from build123d import *

# Parameters (mm, degrees)
F0_R     = 1.5
F0_R_2   = 19
F0_R_3   = 17.5
F1_DEPTH = 2
F2_SIZE  = 1
F3_SIZE  = 1.5


with BuildPart() as f1:
    # F0 (on Top) → F1 (new body)
    with BuildSketch(Plane.XY):
        with BuildLine():
            Line((-22.3, 19.5), (-22.3, -19.5))
            ThreePointArc((-22.3, -19.5), (-21.4798989873, -21.4798989873), (-19.5, -22.3))
            Line((-19.5, -22.3), (19.5, -22.3))
            ThreePointArc((19.5, -22.3), (21.4798989873, -21.4798989873), (22.3, -19.5))
            Line((22.3, -19.5), (22.3, 19.5))
            ThreePointArc((22.3, 19.5), (21.4798989873, 21.4798989873), (19.5, 22.3))
            Line((19.5, 22.3), (-19.5, 22.3))
            ThreePointArc((-19.5, 22.3), (-21.4798989873, 21.4798989873), (-22.3, 19.5))
        make_face()
        with Locations((-19.5, -19.5)):
            Circle(F0_R, mode=Mode.SUBTRACT)
        with Locations((19.5, -19.5)):
            Circle(F0_R, mode=Mode.SUBTRACT)
        with Locations((-19.5, 19.5)):
            Circle(F0_R, mode=Mode.SUBTRACT)
        Circle(F0_R_2, mode=Mode.SUBTRACT)
        with Locations((19.5, 19.5)):
            Circle(F0_R, mode=Mode.SUBTRACT)
        Circle(F0_R_2)
        Circle(F0_R_3, mode=Mode.SUBTRACT)
    extrude(amount=F1_DEPTH)

    # F2
    f2_edges = [f1.edges().sort_by_distance(p)[0] for p in [
        (-21, 19.5, 2),
        (18, 19.5, 2),
        (18, -19.5, 2),
        (-21, -19.5, 2),
    ]]
    chamfer(f2_edges, length=F2_SIZE)

    # F3
    f3_edges = [f1.edges().sort_by_distance(p)[0] for p in [
        (-17.5, 0, 0),
    ]]
    chamfer(f3_edges, length=F3_SIZE)


solid = f1.part
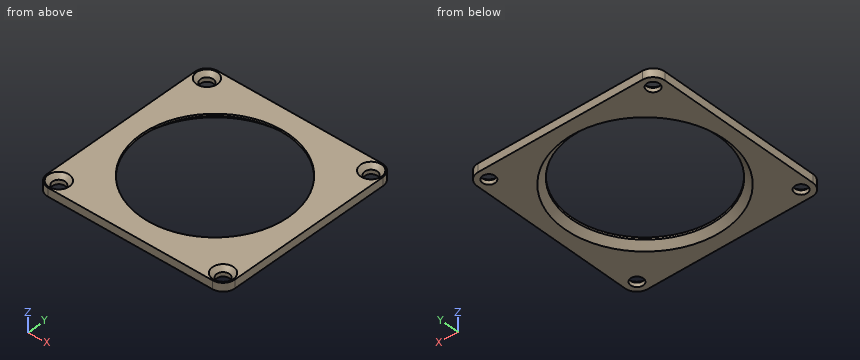
For this review, take the finished solid that the model builds, in its own axes (mm). Coordinates: 2 decimals unless noted, no trailing zeros. Loops run counter-clockwise (first coordinate to the right, second up) from the corner with the lowest first, then second, coordinate; pieces in that order, holes last. Notation, with made-up numbers: (-19, 8) - (-2, 8) arc R30 ccw to (-2, 33) - close; hole circle Ø3 at (22, 51.25). An arc over 180 degrees is marked (long way). Use a Markdown table: item, result. Add a question column.
Item 1: We need section A-A (x = 0). Give the boundary of the cut face in (y, z).
Item 2: For line 1 (Y direction, x = 19.5, z = 0.45); line 2 (Y direction, x = 0, z = 1.8); line 3 (Y direction, x = 19.5, z = 1.8), list the stretches that pass through material, from the lowest coordinate up.
Item 3: Insertion check: pin 1 Ø3.5 at (x, y) = (19.5, 19.5) entering from +Z; pin 2 Ø2.5 at (x, y) = (-19.5, -19.5) entering from -Z. Each pin has a flat end and moves straight along its axis. Give the tip position at first contact, or say it passes through.
Results list:
| question | item | result |
|---|---|---|
| 1 | outline | (-22.3, 0) - (-19, 0) - (-17.5, 1.5) - (-17.5, 2) - (-22.3, 2) - close; (17.5, 1.5) - (19, 0) - (22.3, 0) - (22.3, 2) - (17.5, 2) - close |
| 2 | line 1 | y = -22.3 to -21, -18 to 18, 21 to 22.3 |
| 2 | line 2 | y = -22.3 to -17.5, 17.5 to 22.3 |
| 2 | line 3 | y = -22.3 to -21.8, -17.2 to 17.2, 21.8 to 22.3 |
| 3 | pin 1 | stops at z = 1.25 |
| 3 | pin 2 | passes through |
